```python
from build123d import *

# Parameters (mm, degrees)
SKETCH1_W           = 5.5
SKETCH1_H           = 5.5
BOSS_EXTRUDE1_DEPTH = 35
SKETCH3_R           = 1.5
CUT_EXTRUDE1_DEPTH  = 10


with BuildPart() as part:
    # Sketch1 → Boss-Extrude1 (new, symmetric)
    with BuildSketch(Plane(origin=(0, 0, 0), x_dir=(1, 0, 0), z_dir=(0, 1, 0))):
        Rectangle(SKETCH1_W, SKETCH1_H)
    extrude(amount=BOSS_EXTRUDE1_DEPTH, both=True)

    # Sketch3 → Cut-Extrude1 (cut)
    with BuildSketch(Plane(origin=(0, 35, 0), x_dir=(1, 0, 0), z_dir=(0, 1, 0))):
        with Locations(Location((0, 0, 0), (0, 0, 270))):
            Circle(SKETCH3_R)
    cut_extrude1 = extrude(amount=-CUT_EXTRUDE1_DEPTH, mode=Mode.SUBTRACT)

    # Mirror1: Cut-Extrude1 across plane
    add(cut_extrude1.mirror(Plane.ZX), mode=Mode.SUBTRACT)


solid = part.part
```
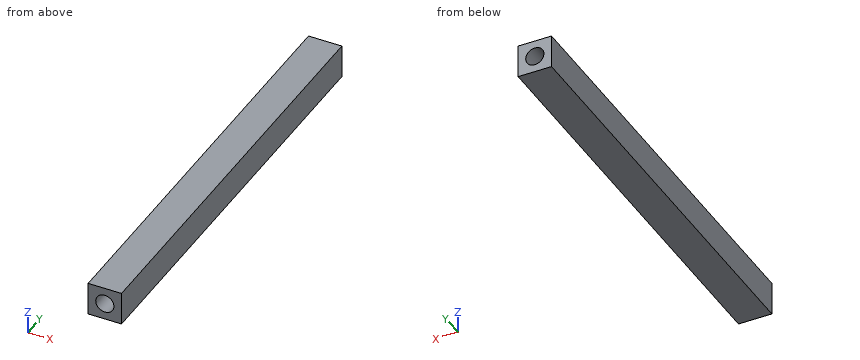
Can you work these out from the model? Positions are in its coordinate system, mm. Give positions to 0.01 mm unless a question says otherwise; leave off trailing zeros. Write each loop counter-clockwise with the first axis right and the second up, starting at its lowest first coordinate (ties: lowest second). Pieces come first, ordered by that corner, then holes. Notation, with made-up numbers: (42, -21.75) - (100, -21.75) arc R24 cw to (100, 7.25) - close; hole circle Ø1 at (76.5, 31). An arc over 180 degrees is marked (long way). Write item = value, one per line. Start each with the question number.
1. Imagine slicing it at A-A (z = 0). Please give me the cut outline in (x, y), and give its area (3 significant figures).
2. For pin 1 (2.5 mm diameter, centred on x = 0, z = 0, fed in from +Y), with a flat end and sliding along its axis, tell me the tip position at first contact or that it passes through.
3. Please list where these lines run through material, in increasing order: line 1 (X direction, y = -30.5, z = 0); line 2 (Y direction, x = -0.6, z = -0.7); line 3 (Z direction, x = 1.15, y = 26).
4. Imagine slicing it at B-B (x = 0). Please give me the cut outline in (y, z).
Worked answers:
q1.outline = (-2.75, -35) - (-1.5, -35) - (-1.5, -25) - (1.5, -25) - (1.5, -35) - (2.75, -35) - (2.75, 35) - (1.5, 35) - (1.5, 25) - (-1.5, 25) - (-1.5, 35) - (-2.75, 35) - close
q1.area = 325 mm2
q2.pin_1 = 25
q3.line_1 = -2.75 to -1.5, 1.5 to 2.75
q3.line_2 = -25 to 25
q3.line_3 = -2.75 to -0.96, 0.96 to 2.75
q4.outline = (-35, -2.75) - (35, -2.75) - (35, -1.5) - (25, -1.5) - (25, 1.5) - (35, 1.5) - (35, 2.75) - (-35, 2.75) - (-35, 1.5) - (-25, 1.5) - (-25, -1.5) - (-35, -1.5) - close
